Work out the finished part from the listing and answer in its coordinate system (mm). A direction names the side the tool comes from. Give positions to 0.01 mm unless a question says otherwise; leave off trailing zeros. Loops run counter-clockwise (first coordinate to the right, second up) from the corner with the lowest first, then second, coordinate; pieces in that order, holes last. Notation, with made-up numbers: (15.5, -3) - (29.5, -3) arc R12 cw to (29.5, 18) - close; hole circle Ø4 at (4, 53.5). An arc over 180 degrees is marked (long way). Use one line per item in the form item = value. Start each with the question number.
from build123d import *

# Parameters (mm, degrees)
BOTTON_SHAFT_DEPTH = 3.25
SCHIZZO2_R         = 4.5
NUT_BLOCK_DEPTH    = 4
TOP_SHAFT_DEPTH    = 29.5


with BuildPart() as part:
    # Hex-nut-botton → Botton shaft (new, symmetric)
    with BuildSketch(Plane.XY):
        Polygon((11.142860195, 0), (5.571430098, 9.65), (-5.571430098, 9.65), (-11.142860195, 0), (-5.571430098, -9.65), (5.571430098, -9.65), align=None)
        Polygon((7.867433715, 0.473205081), (4.343524479, 6.576794919), (4.170319398, 7.223205081), (3.523909236, 7.05), (-3.523909236, 7.05), (-4.170319398, 7.223205081), (-4.343524479, 6.576794919), (-7.867433715, 0.473205081), (-8.340638796, 0), (-7.867433715, -0.473205081), (-4.343524479, -6.576794919), (-4.170319398, -7.223205081), (-3.523909236, -7.05), (3.523909236, -7.05), (4.170319398, -7.223205081), (4.343524479, -6.576794919), (7.867433715, -0.473205081), (8.340638796, 0), align=None, mode=Mode.SUBTRACT)
    extrude(amount=BOTTON_SHAFT_DEPTH, both=True)

    # Schizzo2 → Nut block (add)
    with BuildSketch(Plane.XY.offset(3.25)):
        Polygon((5.571430098, 9.65), (-5.571430098, 9.65), (-11.142860195, 0), (-5.571430098, -9.65), (5.571430098, -9.65), (11.142860195, 0), align=None)
        Circle(SCHIZZO2_R, mode=Mode.SUBTRACT)
    extrude(amount=NUT_BLOCK_DEPTH)

    # Hex-nut-top → Top shaft (add)
    with BuildSketch(Plane.XY.offset(7.25)):
        Polygon((11.142860195, 0), (5.571430098, 9.65), (-5.571430098, 9.65), (-11.142860195, 0), (-5.571430098, -9.65), (5.571430098, -9.65), align=None)
        Polygon((7.867433715, 0.473205081), (4.343524479, 6.576794919), (4.170319398, 7.223205081), (3.523909236, 7.05), (-3.523909236, 7.05), (-4.170319398, 7.223205081), (-4.343524479, 6.576794919), (-7.867433715, 0.473205081), (-8.340638796, 0), (-7.867433715, -0.473205081), (-4.343524479, -6.576794919), (-4.170319398, -7.223205081), (-3.523909236, -7.05), (3.523909236, -7.05), (4.170319398, -7.223205081), (4.343524479, -6.576794919), (7.867433715, -0.473205081), (8.340638796, 0), align=None, mode=Mode.SUBTRACT)
    extrude(amount=TOP_SHAFT_DEPTH)


solid = part.part
1) A cutting plane is placed at C-C (z = 29). Give the vertices of the cut face in (x, y).
2) A cutting plane is placed at A-A (x = 0). Give the vertices of the cut face in (y, z).
3) Find the intervals of material crossed by probe 1 along Y at (x, z) = (0, 5.7); probe 2 along Y at (x, z) = (-0.5, 24.5); probe 3 along Z at (x, y) = (-5.5, 1.75), in increasing order.
4) A tool of negligible diameter and unlimited length cuts with its end or side. For faces 1 (the flat face through (7, -3, -3.25)), 2 (the flat face through (6.08, -3.57, 21.79)), 3 (the flat face through (6.08, -3.57, 0.05)), from which of +Z, -Z, +X, -X, +Y, -Y can it reach the whole face along a straight path? Write none if from no direction.
5) Flat-ended cylindrical pins translate along their axes: pin 1 Ø7 at (x, y) = (1.5, 3) entering from +Z; pin 2 Ø5 at (y, z) = (-6.5, 7.5) entering from +X. Find the tip coordinate at first contact, or state that the pin passes through.
6) A cutting plane is placed at D-D (x = -6). Give the vertices of the cut face in (y, z), plus the area to 3 significant figures.
7) A cutting plane is placed at B-B (y = -1.25). Give the vertices of the cut face in (x, z).
Answer sheet:
q1.outline = (-11.14, 0) - (-5.57, -9.65) - (5.57, -9.65) - (11.14, 0) - (5.57, 9.65) - (-5.57, 9.65) - close; hole (-8.34, 0) - (-7.87, -0.47) - (-4.34, -6.58) - (-4.17, -7.22) - (-3.52, -7.05) - (3.52, -7.05) - (4.17, -7.22) - (4.34, -6.58) - (7.87, -0.47) - (8.34, 0) - (7.87, 0.47) - (4.34, 6.58) - (4.17, 7.22) - (3.52, 7.05) - (-3.52, 7.05) - (-4.17, 7.22) - (-4.34, 6.58) - (-7.87, 0.47) - close
q2.outline = (-9.65, -3.25) - (-7.05, -3.25) - (-7.05, 3.25) - (-4.5, 3.25) - (-4.5, 7.25) - (-7.05, 7.25) - (-7.05, 36.75) - (-9.65, 36.75) - close; (4.5, 3.25) - (7.05, 3.25) - (7.05, -3.25) - (9.65, -3.25) - (9.65, 36.75) - (7.05, 36.75) - (7.05, 7.25) - (4.5, 7.25) - close
q3.probe_1 = -9.65 to -4.5, 4.5 to 9.65
q3.probe_2 = -9.65 to -7.05, 7.05 to 9.65
q3.probe_3 = 3.25 to 7.25
q4.face_1 = -Z, +X, -X, +Y, -Y
q4.face_2 = +Z
q4.face_3 = -Z
q5.pin_1 = 7.25
q5.pin_2 = 8.83
q6.outline = (-8.91, -3.25) - (-3.71, -3.25) - (-3.71, 3.25) - (3.71, 3.25) - (3.71, -3.25) - (8.91, -3.25) - (8.91, 36.75) - (3.71, 36.75) - (3.71, 7.25) - (-3.71, 7.25) - (-3.71, 36.75) - (-8.91, 36.75) - close
q6.area = 446 mm²
q7.outline = (-10.42, -3.25) - (-7.42, -3.25) - (-7.42, 3.25) - (-4.32, 3.25) - (-4.32, 7.25) - (-7.42, 7.25) - (-7.42, 36.75) - (-10.42, 36.75) - close; (4.32, 3.25) - (7.42, 3.25) - (7.42, -3.25) - (10.42, -3.25) - (10.42, 36.75) - (7.42, 36.75) - (7.42, 7.25) - (4.32, 7.25) - close
